The model under review builds one solid part; all positions refer to its coordinate system, in mm. Face numbers are marked on the shaded views. A direction names the side the tool comes from. Round coordinates to 2 decimals unless told otherwise and drop trailing zeros.
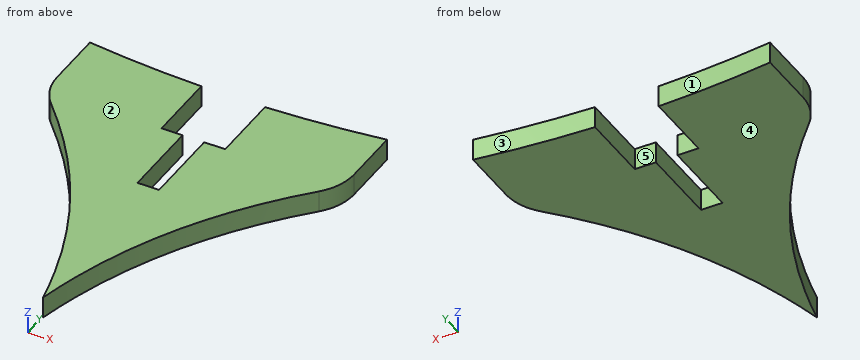
```python
from build123d import *

# Parameters (mm, degrees)
BOSS_EXTRU_1_DEPTH = 4
CONG_1_R           = 10


with BuildPart() as part:
    # Esquisse1 → Boss.-Extru.1 (new body)
    with BuildSketch(Plane.XY):
        with BuildLine():
            Line((-27.5, 32.5), (-27.5, 17.5))
            add(Edge.make_bspline(
                [(-27.5, 17.5), (-6.129432255, -3.700842112), (0, -32.5)],
                knots=[0, 0, 0, 1, 1, 1], degree=2))
            add(Edge.make_bspline(
                [(27.5, 17.5), (6.129432255, -3.700842112), (0, -32.5)],
                knots=[0, 0, 0, 1, 1, 1], degree=2))
            Line((27.5, 17.5), (27.5, 32.5))
            ThreePointArc((27.5, 32.5), (16.723379615, 31.330378268), (5.9, 30.732034209))
            Line((5.9, 30.732034209), (5.9, 17.5))
            Line((5.9, 17.5), (2, 17.5))
            Line((2, 17.5), (2, 2.5))
            Line((2, 2.5), (-2, 2.5))
            Line((-2, 2.5), (-2, 17.5))
            Line((-2, 17.5), (-5.9, 17.5))
            Line((-5.9, 17.5), (-5.9, 30.732034209))
            ThreePointArc((-5.9, 30.732034209), (-16.723379615, 31.330378268), (-27.5, 32.5))
        make_face()
    extrude(amount=BOSS_EXTRU_1_DEPTH)

    # Congé1
    cong_1_edges = [part.edges().sort_by_distance(p)[0] for p in [
        (-27.5, 17.5, 2),
        (27.5, 17.5, 2),
    ]]
    fillet(cong_1_edges, radius=CONG_1_R)


solid = part.part
```
(1) For the marked faces 1 and 2, list the 3-axis set-ups (+Z, -Z, +X, -X, +Y, -Y) from which the entire face can be reached by the end or side of a thin tool; tool diameter is ignored.
Data:
face 1: +Z, -Z, +Y
face 2: +Z, +X, -X, +Y, -Y
(2) Draft analysis for pull direction X (two halves, no side actions). For the marked faces 3, 4 and 5, state which applies: pulls with the +X half, pulls with the -X half, needs draft (parallel to the pull), parting line crosses it, or undercut.
Data:
face 3: undercut
face 4: needs draft
face 5: undercut
(3) To check wall thickness, follow probe 1 along X at (y, z) = (27, 2); probe 2 along Y at (x, z) = (16.5, 2.6); probe 3 along X at (y, z) = (-10, 2.95). State the ranges of each line that lie inside material, in increasing order.
Data:
probe 1: x = -27.5 to -5.9, 5.9 to 27.5
probe 2: y = 4.72 to 31.31
probe 3: x = -7.67 to 7.67
(4) Insertion check: pin 1 (2 mm diameter, centred on x = -3.5, z = 1.5, fed in from +Y); pin 2 (2 mm diameter, centred on x = 0, z = 2, fed in from +Y); pin 3 (1.5 mm diameter, centred on x = -10.5, z = 3, fed in from -Y). Each pin has a flat end and moves straight along its axis. Give the tip position at first contact, or say it passes through.
Data:
pin 1: stops at y = 17.5
pin 2: stops at y = 2.5
pin 3: stops at y = -5.95
